Model file for the job. Use its own axes, mm. Face numbers are marked on the shaded views. A direction names the side the tool comes from. Round coordinates to 2 decimals unless told otherwise and drop trailing zeros. Order: outer loops, then holes, each group sorted by start corner. A loop starts at its lowest first (then second) coordinate and runs counter-clockwise, first axis right, second up. Notation, with made-up numbers: (42, 9.25) -> (46, 9.25) arc R26 cw to (46, 47.25) -> close; hole circle Ø1 at (66.5, -38.75). An arc over 180 degrees is marked (long way). Answer as CSV lines item,"result".
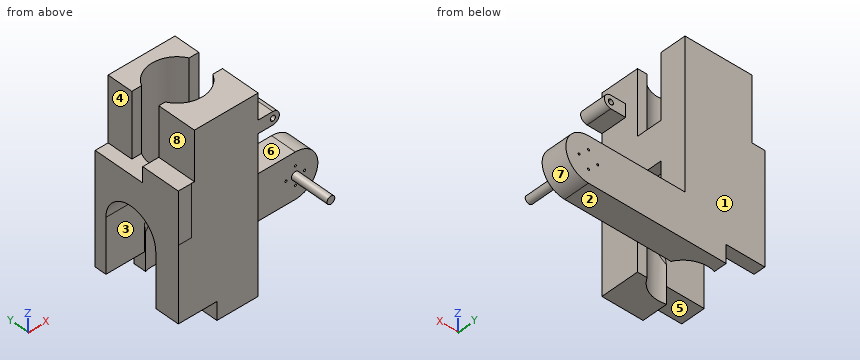
```python
from build123d import *

# Parameters (mm, degrees)
EXTRUDE_1_DEPTH          = 140
EXTRUDE_1_DEPTH_BACK     = 10
SKETCH_2_W               = 52
SKETCH_2_H               = 70
SKETCH_3_W               = 94.267280548
SKETCH_3_H               = 20
CUT_EXTRUDE_1_DEPTH      = 50
SKETCH_4_W               = 2.5
SKETCH_4_H               = 30
CUT_EXTRUDE_2_DEPTH      = 38
EXTRUDE_2_DEPTH          = 20
CUT_EXTRUDE_7_DEPTH      = 152.678113121
CUT_EXTRUDE_7_DEPTH_BACK = 152.678113121
SKETCH_12_R              = 21
SKETCH_14_W              = 100
SKETCH_14_H              = 20
CUT_EXTRUDE_10_DEPTH     = 10
SKETCH_15_W              = 10
SKETCH_15_H              = 70
EXTRUDE_3_DEPTH          = 100
SKETCH_16_W              = 10
SKETCH_16_H              = 30
EXTRUDE_4_DEPTH          = 92
SKETCH_17_R              = 21
CUT_EXTRUDE_11_DEPTH     = 35
SKETCH_20_W              = 14
SKETCH_20_H              = 19
SKETCH_20_H_2            = 42
SKETCH_20_H_3            = 9
SKETCH_20_W_2            = 21
CUT_EXTRUDE_15_DEPTH     = 30
EXTRUDE_5_DEPTH          = 40
SKETCH_23_R              = 21
CUT_EXTRUDE_16_DEPTH     = 35
SKETCH_24_W              = 30
SKETCH_24_H              = 20
EXTRUDE_6_DEPTH          = 8
SKETCH_25_W              = 35
SKETCH_25_H              = 20
EXTRUDE_7_DEPTH          = 75
SKETCH_26_R              = 17.5
EXTRUDE_8_DEPTH          = 20
SKETCH_27_R              = 3
EXTRUDE_9_DEPTH          = 50
M2X0_4_1_D               = 1.6


with BuildPart() as part:
    # ｽｹｯﾁ2 → ﾎﾞｽ - 押し出し1 (new, two sides: drawn at the far end of the back side and taken through both)
    with BuildSketch(Plane.XY.offset(-EXTRUDE_1_DEPTH_BACK)):
        with Locations((0, -5)):
            Rectangle(SKETCH_2_W, SKETCH_2_H)
    extrude(amount=EXTRUDE_1_DEPTH + EXTRUDE_1_DEPTH_BACK)

    # ｽｹｯﾁ3 → ｶｯﾄ - 押し出し1 (cut)
    with BuildSketch(Plane.XY.offset(140)):
        Rectangle(SKETCH_3_W, SKETCH_3_H)
    extrude(amount=-CUT_EXTRUDE_1_DEPTH, mode=Mode.SUBTRACT)

    # ｽｹｯﾁ4 → ｶｯﾄ - 押し出し2 (cut)
    with BuildSketch(Plane.XY.offset(140)):
        with Locations((-24.75, -25)):
            Rectangle(SKETCH_4_W, SKETCH_4_H)
    extrude(amount=-CUT_EXTRUDE_2_DEPTH, mode=Mode.SUBTRACT)

    # ｽｹｯﾁ6 → ﾎﾞｽ - 押し出し2 (add)
    with BuildSketch(Plane(origin=(0, -40, 0), x_dir=(-1, 0, 0), z_dir=(0, -1, 0))):
        with BuildLine():
            Line((-37.5, -120), (-26, -120))
            Line((-26, -120), (-26, -110))
            Line((-26, -110), (-37.5, -110))
            ThreePointArc((-37.5, -110), (-33.964466094, -111.464466094), (-32.5, -115))
            ThreePointArc((-32.5, -115), (-33.964466094, -118.535533906), (-37.5, -120))
        make_face()
        with BuildLine():
            ThreePointArc((-37.5, -110), (-42.5, -115), (-37.5, -120))
            Line((-37.5, -120), (-37.5, -117))
            ThreePointArc((-37.5, -117), (-39.5, -115), (-37.5, -113))
            Line((-37.5, -113), (-37.5, -110))
        make_face()
        with BuildLine():
            Line((-37.5, -117), (-37.5, -120))
            ThreePointArc((-37.5, -120), (-33.964466094, -118.535533906), (-32.5, -115))
            ThreePointArc((-32.5, -115), (-33.964466094, -111.464466094), (-37.5, -110))
            Line((-37.5, -110), (-37.5, -113))
            ThreePointArc((-37.5, -113), (-36.085786438, -113.585786438), (-35.5, -115))
            ThreePointArc((-35.5, -115), (-36.085786438, -116.414213562), (-37.5, -117))
        make_face()
    extrude(amount=-EXTRUDE_2_DEPTH)

    # ｽｹｯﾁ12 → ｶｯﾄ - 押し出し7 (cut, two sides: drawn at the far end of the back side and taken through both)
    with BuildSketch(Plane.XY.offset(-CUT_EXTRUDE_7_DEPTH_BACK)):
        Circle(SKETCH_12_R)
    extrude(amount=CUT_EXTRUDE_7_DEPTH + CUT_EXTRUDE_7_DEPTH_BACK, mode=Mode.SUBTRACT)

    # ｽｹｯﾁ14 → ｶｯﾄ - 押し出し10 (cut)
    with BuildSketch(Plane(origin=(26, 0, 0), x_dir=(0, 0, -1), z_dir=(1, 0, 0))):
        with Locations((-40, 0)):
            Rectangle(SKETCH_14_W, SKETCH_14_H)
    extrude(amount=-CUT_EXTRUDE_10_DEPTH, mode=Mode.SUBTRACT)

    # ｽｹｯﾁ15 → ﾎﾞｽ - 押し出し3 (add)
    with BuildSketch(Plane(origin=(0, 0, -10), x_dir=(-1, 0, 0), z_dir=(0, 0, -1))):
        with Locations((31, -5)):
            Rectangle(SKETCH_15_W, SKETCH_15_H)
    extrude(amount=-EXTRUDE_3_DEPTH)

    # ｽｹｯﾁ16 → ﾎﾞｽ - 押し出し4 (add)
    with BuildSketch(Plane(origin=(0, 0, -10), x_dir=(-1, 0, 0), z_dir=(0, 0, -1))):
        with Locations((31, -25)):
            Rectangle(SKETCH_16_W, SKETCH_16_H)
    extrude(amount=-EXTRUDE_4_DEPTH)

    # ｽｹｯﾁ17 → ｶｯﾄ - 押し出し11 (cut)
    with BuildSketch(Plane.ZY.offset(36)):
        with Locations(Location((25, 0, 0), (0, 0, 270))):
            Circle(SKETCH_17_R)
    extrude(amount=-CUT_EXTRUDE_11_DEPTH, mode=Mode.SUBTRACT)

    # ｽｹｯﾁ20 → ｶｯﾄ - 押し出し15 (cut)
    with BuildSketch(Plane.ZY.offset(36)):
        with Locations((-3, -30.5)):
            Rectangle(SKETCH_20_W, SKETCH_20_H)
        with Locations((-3, 0)):
            Rectangle(SKETCH_20_W, SKETCH_20_H_2)
        with Locations((-3, 25.5)):
            Rectangle(SKETCH_20_W, SKETCH_20_H_3)
        with Locations((14.5, 0)):
            Rectangle(SKETCH_20_W_2, SKETCH_20_H_2)
    extrude(amount=-CUT_EXTRUDE_15_DEPTH, mode=Mode.SUBTRACT)

    # ｽｹｯﾁ22 → ﾎﾞｽ - 押し出し5 (add)
    with BuildSketch(Plane.XY.offset(102)):
        Polygon((-36, -40), (-26, -40.058181949), (-26, -10), (-36, -10), align=None)
    extrude(amount=-EXTRUDE_5_DEPTH)

    # ｽｹｯﾁ23 → ｶｯﾄ - 押し出し16 (cut)
    with BuildSketch(Plane.ZY.offset(36)):
        with Locations((46, 0)):
            Circle(SKETCH_23_R)
        with BuildLine():
            ThreePointArc((25, -6e-09), (31.150757593, 14.849242403), (46, 21))
            Line((46, 21), (25, 21))
            Line((25, 21), (25, -6e-09))
        make_face()
        with BuildLine():
            ThreePointArc((46, -21), (31.150757597, -14.849242407), (25, -6e-09))
            Line((25, -6e-09), (25, -21))
            Line((25, -21), (46, -21))
        make_face()
    extrude(amount=-CUT_EXTRUDE_16_DEPTH, mode=Mode.SUBTRACT)

    # ｽｹｯﾁ24 → ﾎﾞｽ - 押し出し6 (add)
    with BuildSketch(Plane(origin=(26, 0, 0), x_dir=(0, 0, -1), z_dir=(1, 0, 0))):
        with Locations((-75, 0)):
            Rectangle(SKETCH_24_W, SKETCH_24_H)
    extrude(amount=-EXTRUDE_6_DEPTH)

    # ｽｹｯﾁ25 → ﾎﾞｽ - 押し出し7 (add)
    with BuildSketch(Plane(origin=(26, 0, 0), x_dir=(0, 0, -1), z_dir=(1, 0, 0))):
        with Locations((-7.5, 20)):
            Rectangle(SKETCH_25_W, SKETCH_25_H)
    extrude(amount=EXTRUDE_7_DEPTH)

    # ｽｹｯﾁ26 → ﾎﾞｽ - 押し出し8 (add)
    with BuildSketch(Plane(origin=(0, 30, 0), x_dir=(1, 0, 0), z_dir=(0, 1, 0))):
        with Locations((101, -7.5)):
            Circle(SKETCH_26_R)
    extrude(amount=-EXTRUDE_8_DEPTH)

    # ｽｹｯﾁ27 → ﾎﾞｽ - 押し出し9 (add)
    with BuildSketch(Plane(origin=(0, 30, 0), x_dir=(1, 0, 0), z_dir=(0, 1, 0))):
        with Locations(Location((101, -7.5, 0), (0, 0, 270))):
            Circle(SKETCH_27_R)
    extrude(amount=-EXTRUDE_9_DEPTH)

    # M2x0.4 ねじ穴1 (through all)
    with Locations(Plane(origin=(0, 30, 0), x_dir=(1, 0, 0), z_dir=(0, 1, 0))):
        with Locations((101, -0.3), (101, -14.7), (108.2, -7.5), (93.8, -7.5)):
            Hole(M2X0_4_1_D / 2)


solid = part.part
```
Q1. Wall check: L1, parallel to Z at x = 101, y = 19; L2, parallel to Y at x = -18, z = 41; L3, parallel to Y at x = 34.5, z = 21. Give the ranges that are in metal, low to high. Write a range as [from, to].
Checks:
L1,"[-10, -0.5], [1.1, 13.9], [15.5, 25]"
L2,"[-40, -21], [21, 30]"
L3,"[10, 30]"
Q2. Flat gauge pins, fed straight in: pin 1 (9 mm diameter, centred on y = -19, z = 122.5, fed in from -X); pin 2 (4 mm diameter, centred on x = 22.5, y = 1, fed in from -Z); pin 3 (4 mm diameter, centred on y = 1, z = 10, fed in from +X); pin 4 (22 mm diameter, centred on y = -33.5, z = 1.5, fed in from -X). Where does each tip first touch, or does it go through?
Checks:
pin 1,"x = -23.5"
pin 2,"z = 60"
pin 3,"x = 103.96"
pin 4,"x = -36"
Q3. Tool access for the marked faces 4, 5, 6, 7 and 8: list every direction of +Z, -Z, +X, -X, +Y, -Y with a clear straight run to the whole face (end or side of a thin tool).
Checks:
face 4,"+Z, -X, +Y"
face 5,"-Z, -X, +Y, -Y"
face 6,"+Z, +X, +Y, -Y"
face 7,"+X, +Y, -Y"
face 8,"+Z, -X, -Y"
Q4. Saw through at B-B (y = 16.5). Write the cut outline in (x, z).
Checks:
outline,"(-36, 58.99) -> (-12.99, 58.99) -> (-12.99, 140) -> (-26, 140) -> (-26, 90) -> (-36, 90) -> close; (12.99, -10) -> (101, -10) arc R17.5 ccw to (101, 25) -> (26, 25) -> (26, 140) -> (12.99, 140) -> close; hole circle Ø1.6 at (93.8, 7.5); hole circle Ø1.6 at (101, 0.3); hole circle Ø1.6 at (101, 14.7); hole circle Ø1.6 at (108.2, 7.5)"
Q5. Saw through at D-D (y = -27.5). Write the cut outline in (x, z), plus the area to 3 significant figures.
Checks:
outline,"(-36, 4) -> (-6, 4) -> (-6, -10) -> (26, -10) -> (26, 110) -> (37.5, 110) arc R5 ccw to (37.5, 120) -> (26, 120) -> (26, 140) -> (-23.5, 140) -> (-23.5, 102) -> (-36, 102) -> close; hole circle Ø4 at (37.5, 115)"
area,"8,550 mm²"
Q6. Saw through at A-A (y = 0). Write the cut outline in (x, z).
Checks:
outline,"(-36, 67) -> (-21, 67) -> (-21, 90) -> (-36, 90) -> close; (18, 60) -> (26, 60) -> (26, 90) -> (18, 90) -> close; circle Ø6 at (101, 7.5)"
Q7. Mould opens along Y. For the marked faces 1, 2 and 3 say: +Y half, -Y half, draft (parallel to the pull), parting line (faces both ways), or undercut.
Checks:
face 1,"+Y half"
face 2,"draft"
face 3,"undercut"
Q8. Saw through at C-C (x = -14). Write the cut outline in (y, z), plus the area to 3 significant figures.
Checks:
outline,"(-40, 4) -> (-21, 4) -> (-21, 46) arc R21 cw to (-15.65, 60) -> (-15.65, 140) -> (-40, 140) -> close; (15.65, 60) arc R21 cw to (21, 46) -> (21, 4) -> (30, 4) -> (30, 140) -> (15.65, 140) -> close"
area,"4,710 mm²"
